The listing builds one solid part. Answer for the finished solid, in the listing's coordinates (mm). Give positions to 0.01 mm unless a question says otherwise; leave off trailing zeros. Order: outer loops, then holes, each group sorted by start corner. A loop starts at its lowest first (then second) coordinate and runs counter-clockwise, first axis right, second up. Notation, with made-up numbers: (14.5, 43) - (33.5, 43) arc R7 cw to (33.5, 51) - close; hole circle Ø8 at (5, 11.25). An arc over 180 degrees is marked (long way). Use CSV: the item, a comma, the result in double quotes.
```python
from build123d import *

# Parameters (mm, degrees)
BOSS_EXTRUDE1_DEPTH = 3
SKETCH2_R           = 34
CUT_EXTRUDE2_DEPTH  = 12
FILLET1_R           = 15


with BuildPart() as part:
    # Sketch1 → Boss-Extrude1 (new body)
    with BuildSketch(Plane(origin=(0, 0, 0), x_dir=(1, 0, 0), z_dir=(0, 1, 0))):
        Polygon((85, 90), (85, 100), (-85, 100), (-85, 90), (-96.461253746, 25), (-66.461253746, 25), (-66.461253746, 0), (66.461253746, 0), (66.461253746, 25), (96.461253746, 25), align=None)
    extrude(amount=BOSS_EXTRUDE1_DEPTH)

    # Sketch2 → Cut-Extrude2 (cut)
    with BuildSketch(Plane(origin=(0, 3, 0), x_dir=(1, 0, 0), z_dir=(0, 1, 0))):
        with Locations(Location((0, 55, 0), (0, 0, 270))):
            Circle(SKETCH2_R)
    extrude(amount=-CUT_EXTRUDE2_DEPTH, mode=Mode.SUBTRACT)

    # Fillet1
    fillet1_edges = [part.edges().sort_by_distance(p)[0] for p in [
        (-96.461253746, 1.5, -25),
        (96.461253746, 1.5, -25),
    ]]
    fillet(fillet1_edges, radius=FILLET1_R)


solid = part.part
```
Item 1: The part is cut by section A-A (x = 0). Give the vertices of the cut face in (y, z).
Taken from the geometry:
outline,"(0, -100) - (3, -100) - (3, -89) - (0, -89) - close; (0, -21) - (3, -21) - (3, 0) - (0, 0) - close"
Item 2: The part is cut by section B-B (y = 0.6). Give the vertices of the cut face in (x, z).
Taken from the geometry:
outline,"(-93.36, -42.6) - (-85, -90) - (-85, -100) - (85, -100) - (85, -90) - (93.36, -42.6) arc R15 ccw to (78.58, -25) - (66.46, -25) - (66.46, 0) - (-66.46, 0) - (-66.46, -25) - (-78.58, -25) arc R15 ccw to start; hole circle Ø68 at (0, -55)"
Item 3: Each of these flat-tipped pins is pushed along its axis until it touches: pin 1 (0.9 mm diameter, centred on x = 72.5, y = 2, fed in from +Z); pin 2 (0.9 mm diameter, centred on y = 2, z = -97, fed in from -X); pin 3 (1 mm diameter, centred on y = 1, z = -13.5, fed in from +X). Where does it stop, or does it pass through?
Taken from the geometry:
pin 1,"z = -25"
pin 2,"x = -85"
pin 3,"x = 66.46"
Item 4: The mould has two halves that part along X. Classify faces 1 (the face through (22.98, 1.52, -80.06)), 2 (the face through (89.237, 1.479, -65.971)), 3 (the face through (-89.12, 1.48, -66.63)): +X half, -X half, draft (parallel to the pull), parting line (faces both ways), or undercut.
Taken from the geometry:
face 1,"undercut"
face 2,"+X half"
face 3,"-X half"
Item 5: Find the intervals of material crossed by line 1 along X through (y, z) = (0.9, -15); line 2 along X through (y, z) = (1.2, -58); line 3 along X through (y, z) = (1.55, -36), in increasing order.
Taken from the geometry:
line 1,"-66.46 to 66.46"
line 2,"-90.64 to -33.87, 33.87 to 90.64"
line 3,"-93.04 to -28.2, 28.2 to 93.04"
Item 6: The part is cut by section C-C (z = -60). Give the vertices of the cut face in (x, y).
Taken from the geometry:
outline,"(-90.29, 0) - (-33.63, 0) - (-33.63, 3) - (-90.29, 3) - close; (33.63, 0) - (90.29, 0) - (90.29, 3) - (33.63, 3) - close"
